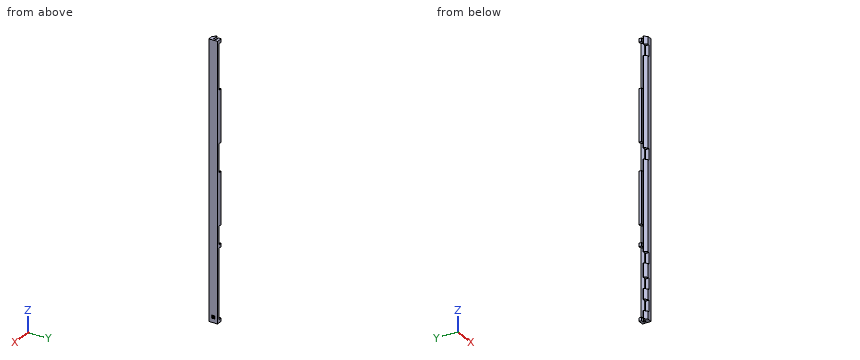
Autodesk Inventor part; units mm, degrees
ref_plane "YZ Plane" through (0, 0, 0) normal (1, 0, 0) x (0, 1, 0)
ref_plane "XZ Plane" through (0, 0, 0) normal (0, 1, 0) x (-1, 0, 0)
ref_plane "XY Plane" through (0, 0, 0) normal (0, 0, 1) x (1, 0, 0)
sketch "Sketch1" plane through (0, 0, 0) normal (0, 0, 1) x (1, 0, 0)
  line L0 (0, 3.75) -> (2, 3.75)
  line L1 (2, 3.75) -> (2, -4)
  line L2 (2, -4) -> (0, -4)
  line L3 (0, -4) -> (0, 3.75) construction
  line L4 (0, -4) -> (-5, -4)
  line L5 (-5, -4) -> (-5, -1)
  line L6 (-5, -1) -> (0, -1)
  line L7 (0, 3.75) -> (-1, 3.75)
  line L8 (-1, 3.75) -> (-1, 0.75)
  line L9 (-1, 0.75) -> (0, 0.75)
  line L10 (0, 0.75) -> (0, 3.75) construction
  line L11 (0, 0.75) -> (0, -1)
  point P0 (0, 0)
  point P1 (0, -0.125)
  point P2 (1, 3.75)
  dimension "d0" = 4
  dimension "d1" = 2
  dimension "d5" = 5
  dimension "d6" = 1.75
  dimension "d7" = 3
  dimension "d11" = 3
  dimension "d12" = 3
extrude "Extrusion1" add sketch "Sketch1" along normal blind 243.25
sketch "Sketch2" plane through (-1, 0.75, 0) normal (-1, 0, 0) x (0, 0, 1)
  line L0 (0, 3) -> (0, 0)
  line L1 (0, 0) -> (243.25, 0)
  line L2 (243.25, 3) -> (243.25, 0)
  line L3 (0, 3) -> (243.25, 3)
  point P0 (0, -0.75)
extrude "Extrusion2" cut sketch "Sketch2" against normal blind 0.9
chamfer "Chamfer1" distance 2.5 angle 45 1 edges at (-5, -4, 121.625)
sketch "Sketch3" plane through (-0.1, 0.75, 0) normal (-1, 0, 0) x (0, 0, 1)
  line L0 (0, 3) -> (243.25, 3)
  line L1 (0, 3) -> (2.95, 3)
  line L2 (2.95, 3) -> (2.95, 0.55)
  line L3 (2.95, 0.55) -> (0, 0.55)
  line L4 (0, 0.55) -> (0, 3)
  line L5 (59.8466, 2.85) -> (59.8466, 0.85) construction
  line L6 (243.25, 3) -> (243.25, 0)
  line L7 (243.25, 3) -> (240.3, 3)
  line L8 (240.3, 3) -> (240.3, 0.55)
  line L9 (240.3, 0.55) -> (243.25, 0.55)
  line L10 (243.25, 0.55) -> (243.25, 3)
  line L11 (200.25, 3) -> (154.25, 3)
  line L12 (154.25, 3) -> (154.25, 0.55)
  line L13 (154.25, 0.55) -> (200.25, 0.55)
  line L14 (200.25, 0.55) -> (200.25, 3)
  line L15 (129.25, 3) -> (83.25, 3)
  line L16 (83.25, 3) -> (83.25, 0.55)
  line L17 (83.25, 0.55) -> (129.25, 0.55)
  line L18 (129.25, 0.55) -> (129.25, 3)
  line L19 (0, 3) -> (243.25, 3)
  line L20 (67.25, 3) -> (64.25, 3)
  line L21 (64.25, 3) -> (64.25, 0.55)
  line L22 (64.25, 0.55) -> (67.25, 0.55)
  line L23 (67.25, 0.55) -> (67.25, 3)
  point P0 (0, -0.75)
  point P1 (59.8466, 3)
  dimension "d18" = 2.45
  dimension "d19" = 2.95
  dimension "d22" = 2.45
  dimension "d23" = 2.95
  dimension "d44" = 43
  dimension "d45" = 160
  dimension "d46" = 114
  dimension "d47" = 89
  dimension "d48" = 176
  dimension "d49" = 179
extrude "Extrusion3" add sketch "Sketch3" along normal blind 2.95
sketch "Sketch4" plane through (2, -4, 0) normal (0, -1, 0) x (1, 0, 0)
  circle A0 centre (-4.4525, -10.6025) radius 0.725 construction
  line L0 (-3.2, -15.005) -> (-3.2, -1) construction
  line L1 (-4.5, 0) -> (0, 0) construction
  line L2 (-4.5, 243.25) -> (0, 243.25) construction
  circle A1 centre (-10.2025, 230.7475) radius 2.55 construction
  circle A2 centre (-10.1275, 141.3958) radius 2.55 construction
  circle A3 centre (-10.2025, 51.9975) radius 2.55 construction
  circle A4 centre (-10.2025, 29.9975) radius 2.55 construction
  circle A5 centre (-10.2025, 10.9975) radius 2.55 construction
  line L3 (-3.2, 6.8975) -> (-7, 6.8975)
  line L4 (-7, 6.8975) -> (-7, 16.8975)
  line L5 (-7, 16.8975) -> (-3.2, 16.8975)
  line L6 (-3.2, 16.8975) -> (-3.2, 6.8975)
  line L7 (-3.2, 25.8975) -> (-7, 25.8975)
  line L8 (-7, 25.8975) -> (-7, 35.8975)
  line L9 (-7, 35.8975) -> (-3.2, 35.8975)
  line L10 (-3.2, 35.8975) -> (-3.2, 25.8975)
  line L11 (-3.2, 47.8975) -> (-7, 47.8975)
  line L12 (-7, 47.8975) -> (-7, 57.8975)
  line L13 (-7, 57.8975) -> (-3.2, 57.8975)
  line L14 (-3.2, 57.8975) -> (-3.2, 47.8975)
  line L15 (-3.2, 137.2957) -> (-7, 137.2957)
  line L16 (-7, 137.2957) -> (-7, 147.2957)
  line L17 (-7, 147.2957) -> (-3.2, 147.2957)
  line L18 (-3.2, 147.2957) -> (-3.2, 137.2957)
  line L19 (-2.1, 243.25) -> (-2.1, 0)
  line L20 (-2.1, 236.6475) -> (-2.1, 226.6475)
  circle A6 centre (-10.2025, -8.0025) radius 2.55 construction
  circle A7 centre (-5.5025, -3.6025) radius 0.725 construction
  line L21 (-3.2, -12.1025) -> (-10.2025, -12.1025) construction
  line L22 (-10.2025, -12.1025) -> (-10.2025, -2.1025) construction
  line L23 (-10.2025, -2.1025) -> (-3.2, -2.1025) construction
  line L24 (-7, 243.25) -> (-7, 0) construction
  line L25 (-7, 0) -> (-7, 243.25)
  line L26 (-7, 226.6475) -> (-3.2, 226.6475)
  line L27 (-3.2, 226.6475) -> (-3.2, 236.6475)
  line L28 (-3.2, 236.6475) -> (-7, 236.6475)
  line L29 (-7, 236.6475) -> (-7, 226.6475)
  point P0 (-2, 0)
  dimension "d26" = 1.5
  dimension "d27" = 1.5
  dimension "d28" = 4.1
  dimension "d29" = 5.9
  dimension "d30" = 4.1
  dimension "d31" = 5.9
  dimension "d32" = 4.1
  dimension "d33" = 5.9
  dimension "d34" = 4.1
  dimension "d35" = 5.9
  dimension "d36" = 4.1
  dimension "d37" = 5.9
  dimension "d40" = 4.1
  dimension "d41" = 5.9
extrude "Extrusion4" cut sketch "Sketch4" against normal up to surface (3 mm away)
sketch "Sketch5" plane through (2, -4, 0) normal (1, 0, 0) x (0, 0, -1)
  line L0 (-6.5846, 5.3849) -> (-3.2283, 5.3849) construction
  line L1 (-3.2283, 5.3849) -> (-3.2283, 2.3349) construction
  line L2 (-3.2283, 2.3349) -> (-6.5846, 2.3349) construction
  line L3 (-6.5846, 2.3349) -> (-6.5846, 5.3849) construction
  line L4 (-6.2429, 5.3849) -> (-5.8075, 5.3849)
  line L5 (-5.8075, 5.3849) -> (-5.8075, 2.3349)
  line L6 (-5.8075, 2.3349) -> (-6.2429, 2.3349)
  line L7 (-6.2429, 2.3349) -> (-6.2429, 5.3849)
  line L8 (-5.1241, 5.3849) -> (-4.6888, 5.3849)
  line L9 (-4.6888, 5.3849) -> (-4.6888, 2.3349)
  line L10 (-4.6888, 2.3349) -> (-5.1241, 2.3349)
  line L11 (-5.1241, 2.3349) -> (-5.1241, 5.3849)
  line L12 (-4.0053, 5.3849) -> (-3.57, 5.3849)
  line L13 (-3.57, 5.3849) -> (-3.57, 2.3349)
  line L14 (-3.57, 2.3349) -> (-4.0053, 2.3349)
  line L15 (-4.0053, 2.3349) -> (-4.0053, 5.3849)
  point P0 (0, 4)
extrude "Extrusion5" cut sketch "Sketch5" against normal blind 1
equation "\"d22\" = d18"
equation "\"d30\" = d28"
equation "\"d31\" = d29"
equation "\"d32\" = d28"
equation "\"d33\" = d29"
equation "\"d34\" = d28"
equation "\"d35\" = d29"
equation "\"d36\" = d28"
equation "\"d37\" = d29"
equation "\"d40\" = d28"
equation "\"d41\" = d29"
properties part number "Case Rail" material "PET Plastic"
The listing builds one solid part. Answer for the finished solid, in the listing's coordinates (mm). Round coordinates to 2 decimals unless told otherwise and drop trailing zeros. Loops run counter-clockwise (first coordinate to the right, second up) from the corner with the lowest first, then second, coordinate; pieces in that order, holes last.
Q1. Find the intervals of material crossed by line 1 (Z direction, x = -2, y = -2.75); line 2 (Z direction, x = -2.5, y = 2.75); line 3 (X direction, y = -1.25, z = 230.5), in increasing order.
Q2. Section C-C, the plane z = 61.5 is taken. Determine the outline of the cut face in (x, y), then the cut area to 3 significant figures.
Q3. Section B-B, the plane z = 193 is taken. Determine the outline of the cut face in (x, y).
Q4. Section A-A, the plane z = 143.5 is taken. Determine the outline of the cut face in (x, y).
Q5. Given pin 1 Ø3 at (x, y) = (-3.5, 1) entering from -Z; pin 2 Ø2.5 at (y, z) = (-2.5, 141.5) entering from -X; pin 3 Ø2 at (y, z) = (2.5, 104) entering from -X; pin 4 Ø2.5 at (x, z) = (-1.5, 138.5) entering from +Y, each flat-ended and moving along its own axis, determine where each tip first touches the part or whether it passes through.
Completed:
1. line 1: z = 0 to 6.9, 16.9 to 25.9, 35.9 to 47.9, 57.9 to 137.3, 147.3 to 226.65, 236.65 to 243.25
1. line 2: z = 0 to 2.95, 64.25 to 67.25, 83.25 to 129.25, 154.25 to 200.25, 240.3 to 243.25
1. line 3: x = -1.2 to 2
2. outline: (-5, -1.5) - (-2.5, -4) - (2, -4) - (2, 3.75) - (-0.1, 3.75) - (-0.1, 0.75) - (0, 0.75) - (0, -1) - (-5, -1) - close
2. area: 27.7 mm2
3. outline: (-5, -1.5) - (-2.5, -4) - (2, -4) - (2, 3.75) - (-3.05, 3.75) - (-3.05, 1.3) - (-0.1, 1.3) - (-0.1, 0.75) - (0, 0.75) - (0, -1) - (-5, -1) - close
4. outline: (-1.2, -4) - (2, -4) - (2, 3.75) - (-0.1, 3.75) - (-0.1, 0.75) - (0, 0.75) - (0, -1) - (-1.2, -1) - close
5. pin 1: stops at z = 0
5. pin 2: stops at x = -1.2
5. pin 3: stops at x = -3.05
5. pin 4: stops at y = -1
